```python
from build123d import *

# Parameters (mm, degrees)
SKETCH1_R           = 29.095
BOSS_EXTRUDE1_DEPTH = 13.208
SKETCH2_R           = 25.97
BOSS_EXTRUDE2_DEPTH = 42.672
BOSS_EXTRUDE3_START = -12.6
SKETCH3_R           = 2.86
BOSS_EXTRUDE3_DEPTH = 12.6
SKETCH4_R           = 4
BOSS_EXTRUDE4_DEPTH = 16.49
BOSS_EXTRUDE5_DEPTH = 10.541
BOSS_EXTRUDE6_START = -46.482
BOSS_EXTRUDE6_DEPTH = 32.639


with BuildPart() as part:
    # Sketch1 → Boss-Extrude1 (new body)
    with BuildSketch(Plane(origin=(0, 0, 0), x_dir=(1, 0, 0), z_dir=(0, 1, 0))):
        with Locations(Location((0, 0, 0), (0, 0, 270))):
            Circle(SKETCH1_R)
    extrude(amount=-BOSS_EXTRUDE1_DEPTH)

    # Sketch2 → Boss-Extrude2 (add)
    with BuildSketch(Plane.XZ.offset(13.208)):
        with Locations(Location((0, 0, 0), (0, 0, 90))):
            Circle(SKETCH2_R)
    extrude(amount=BOSS_EXTRUDE2_DEPTH)

    # Sketch3 → Boss-Extrude3 (add)
    # profile 1 of 2: a face of its own
    with BuildSketch(Plane.XZ.offset(55.88).offset(BOSS_EXTRUDE3_START)):
        with BuildLine():
            Line((37.979011894, -6.582278305), (19.106291889, -17.5895))
            ThreePointArc((19.106291889, -17.5895), (25.97, 0), (19.106291889, 17.5895))
            Line((19.106291889, 17.5895), (37.979011894, 6.582278305))
            ThreePointArc((37.979011894, 6.582278305), (41.76, 0), (37.979011894, -6.582278305))
        make_face()
        with Locations(Location((34.14, 0, 0), (0, 0, 270))):
            Circle(SKETCH3_R, mode=Mode.SUBTRACT)
    # profile 2 of 2: a face of its own
    with BuildSketch(Plane.XZ.offset(55.88).offset(BOSS_EXTRUDE3_START)):
        with BuildLine():
            Line((-37.979011894, 6.582278305), (-19.106291889, 17.5895))
            ThreePointArc((-19.106291889, 17.5895), (-25.97, 0), (-19.106291889, -17.5895))
            Line((-19.106291889, -17.5895), (-37.979011894, -6.582278305))
            ThreePointArc((-37.979011894, -6.582278305), (-41.76, 0), (-37.979011894, 6.582278305))
        make_face()
        with Locations(Location((-34.14, 0, 0), (0, 0, 90))):
            Circle(SKETCH3_R, mode=Mode.SUBTRACT)
    extrude(amount=BOSS_EXTRUDE3_DEPTH)

    # Sketch4 → Boss-Extrude4 (add)
    with BuildSketch(Plane(origin=(0, 0, 0), x_dir=(1, 0, 0), z_dir=(0, 1, 0))):
        with Locations(Location((13.335, 0, 0), (0, 0, 270))):
            Circle(SKETCH4_R)
        with Locations(Location((-13.335, 0, 0), (0, 0, 90))):
            Circle(SKETCH4_R)
    extrude(amount=BOSS_EXTRUDE4_DEPTH)

    # Sketch5 → Boss-Extrude5 (add)
    with BuildSketch(Plane(origin=(0, 0, 0), x_dir=(1, 0, 0), z_dir=(0, 1, 0))):
        with BuildLine():
            Line((-0.762, 10.603000191), (-0.762, -10.603000191))
            ThreePointArc((-0.762, -10.603000191), (0, -11.365), (0.762, -10.603000191))
            Line((0.762, -10.603000191), (0.762, 10.603000191))
            ThreePointArc((0.762, 10.603000191), (0, 11.365), (-0.762, 10.603000191))
        make_face()
    extrude(amount=BOSS_EXTRUDE5_DEPTH)

    # Sketch6 → Boss-Extrude6 (add)
    with BuildSketch(Plane.XZ.offset(55.88).offset(BOSS_EXTRUDE6_START)):
        with BuildLine():
            Line((-19, 39.63), (19, 39.63))
            ThreePointArc((19, 39.63), (20.414213562, 39.044213562), (21, 37.63))
            Line((21, 37.63), (21, 15.278772856))
            ThreePointArc((21, 15.278772856), (0, 25.97), (-21, 15.278772856))
            Line((-21, 15.278772856), (-21, 37.63))
            ThreePointArc((-21, 37.63), (-20.414213562, 39.044213562), (-19, 39.63))
        make_face()
    extrude(amount=BOSS_EXTRUDE6_DEPTH)


solid = part.part
```
Part model, mm, in its own coordinate system. A direction names the side the tool comes from. Coordinates: 2 decimals unless noted, no trailing zeros. Write each loop counter-clockwise with the first axis right and the second up, starting at its lowest first coordinate (ties: lowest second). Pieces come first, ordered by that corner, then holes.
Item 1: Slice it at D-D (z = 16.5). Write the cut outline in (x, y).
Item 2: Pin check, flat tips, straight feed: pin 1 (12 mm diameter, centred on x = 26, z = 26.5, fed in from +Y); pin 2 (9.5 mm diameter, centred on x = 5.5, z = 30, fed in from +Y); pin 3 (6 mm diameter, centred on y = 0, z = 4.5, fed in from -X). Stop position of each tip, or through.
Item 3: Slice it at C-C (x = -34.14). Write the cut outline in (y, z), and give its area (3 significant figures).
Item 4: Mould opens along X. For faces 6 (the face through (0, -25, 39.63)), 7 (the face through (-33.04, -49.49, 2.64)), 8 (the face through (41.76, -49.49, 0.11)), 9 (the face through (-21, -25, 26)) say: released by +X, released by -X, zero draft, split by the parting line, or undercut.
Item 5: Slice it at B-B (y = -49.5). Write the cut outline in (x, z), and give its area (3 significant figures).
Item 6: Probe line 1 (Y direction, x = 25, z = 5); line 2 (Y direction, x = 0, z = -11); line 3 (Y direction, x = -26, z = 4.5). List the from-to ranges inside material, lowest first.
Item 7: Slice it at A-A (z = 0). Count the separate pieces of the cut face and the enclosed holes in it, and give its area (3 significant figures).
Item 8: Which spindle directions (+Z, -Z, +X, -X, +Y, -Y) get a long thin tool onto all of the face, cutting with end or side? Do faces 1 (the face through (9, -13.208, -25)), 2 (the face through (-28.411, -49.492, -12.163)), 3 (the face through (28.67, -49.49, -12.01)), 4 (the face through (-0.762, 5, 0)), 5 (the face through (-6, 0, 0)). Say none if no direction does.
Results found:
1. outline: (-23.96, -13.21) - (-21, -13.21) - (-21, -42.04) - (-20.05, -42.04) - (-20.05, -43.28) - (-20.97, -43.28) - (-20.97, -55.88) - (20.97, -55.88) - (20.97, -43.28) - (20.05, -43.28) - (20.05, -42.04) - (21, -42.04) - (21, -13.21) - (23.96, -13.21) - (23.96, 0) - (-23.96, 0) - close
2. pin 1: stops at y = -9.4
2. pin 2: stops at y = 0
2. pin 3: stops at x = -29.06
3. outline: (-55.88, -8.82) - (-43.28, -8.82) - (-43.28, -2.86) - (-55.88, -2.86) - close; (-55.88, 2.86) - (-43.28, 2.86) - (-43.28, 8.82) - (-55.88, 8.82) - close
3. area: 150 mm2
4. face 6: zero draft
4. face 7: undercut
4. face 8: released by +X
4. face 9: released by -X
5. outline: (-37.98, -6.58) - (-19.11, -17.59) arc R25.97 ccw to (19.11, -17.59) - (37.98, -6.58) arc R7.62 ccw to (37.98, 6.58) - (19.11, 17.59) arc R25.97 ccw to (-19.11, 17.59) - (-37.98, 6.58) arc R7.62 ccw to start; hole circle Ø5.72 at (-34.14, 0); hole circle Ø5.72 at (34.14, 0)
5. area: 2,720 mm2
6. line 1: y = -55.88 to 0
6. line 2: y = -55.88 to 10.54
6. line 3: y = -55.88 to -43.28, -13.21 to 0
7. separate pieces: 3
7. enclosed holes: 0
7. area: 3,520 mm2
8. face 1: none
8. face 2: -Z, -X, -Y
8. face 3: -Z, +X, -Y
8. face 4: +Z, -Z, +Y
8. face 5: +Y
